Build history of the part. All positions in model axes, mm. A direction names the side the tool comes from. Coordinates: 2 decimals unless noted, no trailing zeros. Loops run counter-clockwise (first coordinate to the right, second up) from the corner with the lowest first, then second, coordinate; pieces in that order, holes last.
Item 1: 3-axis set-ups, long thin cutter, end or side, ignore diameter. For faces 5 (the face through (36.42, -54.31, -4.31)), 6 (the face through (-47.44, -54.53, -50.96)), 7 (the face through (45, -52.5, -28)), 8 (the face through (36.42, -54.31, -51.69)), 9 (the face through (-25.3, -54.74, -27.7)): which of +Z, -Z, +X, -X, +Y, -Y reach the whole face in a straight line?
Item 2: Cut at A-A (x = 0). List the corners of the cut face in (y, z).
Item 3: Mould opens along Z. For faces 1 (the face through (2, -1, 5)), 2 (the face through (25.53, -54.81, -27.7)), 3 (the face through (0, -52, -47.5)), 4 (the face through (0, -52, -8.5)) say: released by +Z, released by -Z, zero draft, split by the parting line, or undercut.
Item 4: Drill centre lines: line 1 along Z through (x, y) = (-49.75, -53.45); line 2 along Z through (x, y) = (49, -55); line 3 along Z through (x, y) = (-0.5, -9.5). Where is each one in solid material? Low to high.
Item 5: Cut at C-C (z = -73). List the corners of the cut face in (x, y), and give its area (3 significant figures).
Item 6: Flat gauge pins, fed straight in: pin 1 (1.5 mm diameter, centred on y = -29, z = -39.5, fed in from +X); pin 2 (10 mm diameter, centred on x = 0.5, y = -53, fed in from -Z); pin 3 (10 mm diameter, centred on x = 6, y = -51, fed in from +Z). Where does each tip first touch, or does it go through?
Item 7: Cut at B-B (z = -39). List the corners of the cut face in (x, y), and give its area (3 significant figures).
from build123d import *

# Parameters (mm, degrees)
SKETCH1_R           = 50.5
BOSS_EXTRUDE1_DEPTH = 76
SKETCH2_R           = 4
BOSS_EXTRUDE2_DEPTH = 27.5
SKETCH3_R           = 15.5
BOSS_EXTRUDE3_DEPTH = 56
CUT_EXTRUDE1_DEPTH  = 14
SKETCH6_R           = 50.5
BOSS_EXTRUDE4_DEPTH = 69
CUT_EXTRUDE2_REACH  = 109
SKETCH7_R           = 2.5
CUT_EXTRUDE3_START  = -229.584638372
SKETCH8_W           = 6
SKETCH8_H           = 2
CUT_EXTRUDE3_DEPTH  = 230.584638372
CIRPATTERN1_COUNT   = 2
CIRPATTERN1_ANGLE   = 90


with BuildPart() as part:
    # Sketch1 → Boss-Extrude1 (new body)
    with BuildSketch(Plane.XY):
        Circle(SKETCH1_R)
    extrude(amount=-BOSS_EXTRUDE1_DEPTH)

    # Sketch2 → Boss-Extrude2 (add)
    with BuildSketch(Plane.XY):
        Circle(SKETCH2_R)
    extrude(amount=BOSS_EXTRUDE2_DEPTH)

    # Sketch3 → section 1 of loft1
    with BuildSketch(Plane(origin=(0, 0, -82), x_dir=(-1, 0, 0), z_dir=(0, 0, -1)), mode=Mode.PRIVATE) as loft1_s1:
        Circle(SKETCH3_R)
    # loft from a face of the part (loft1)
    loft([part.faces().sort_by_distance((0, 0, -76))[0], loft1_s1.sketch])

    # Sketch4 → Boss-Extrude3 (add)
    with BuildSketch(Plane.XY):
        with BuildLine():
            Line((-55.75, -52.5), (-33.867548492, -52.5))
            ThreePointArc((-33.867548492, -52.5), (-25.666216724, -50.654640627), (-18.012227442, -47.178487286))
            ThreePointArc((-18.012227442, -47.178487286), (0, -50.5), (18.012227442, -47.178487286))
            ThreePointArc((18.012227442, -47.178487286), (25.666216724, -50.654640627), (33.867548492, -52.5))
            Line((33.867548492, -52.5), (55.75, -52.5))
            ThreePointArc((55.75, -52.5), (57.75, -54.5), (55.75, -56.5))
            Line((55.75, -56.5), (33.635158839, -56.5))
            ThreePointArc((33.635158839, -56.5), (25.41686368, -54.776707383), (17.660730448, -51.559175711))
            ThreePointArc((17.660730448, -51.559175711), (0, -54.5), (-17.660730448, -51.559175711))
            ThreePointArc((-17.660730448, -51.559175711), (-25.41686368, -54.776707383), (-33.635158839, -56.5))
            Line((-33.635158839, -56.5), (-55.75, -56.5))
            ThreePointArc((-55.75, -56.5), (-57.75, -54.5), (-55.75, -52.5))
        make_face()
    extrude(amount=-BOSS_EXTRUDE3_DEPTH)

    # Sketch5 → Cut-Extrude1 (cut)
    with BuildSketch(Plane.XZ.offset(56.5)):
        Polygon((-31, -8.5), (31, -8.5), (42, 0), (-42, 0), align=None)
        Polygon((-42, -56), (-31, -47.5), (31, -47.5), (42, -56), align=None)
    extrude(amount=-CUT_EXTRUDE1_DEPTH, mode=Mode.SUBTRACT)

    # Sketch6 → Boss-Extrude4 (add)
    with BuildSketch(Plane.XY):
        Circle(SKETCH6_R)
    extrude(amount=-BOSS_EXTRUDE4_DEPTH)

    # Sketch7 → Cut-Extrude2 (cut, up to next)
    with BuildSketch(Plane.XZ.offset(56.5), mode=Mode.PRIVATE) as cut_extrude2_sk1:
        with Locations((-49.75, -6)):
            Circle(SKETCH7_R)
    cut_extrude2_tool1 = extrude(cut_extrude2_sk1.sketch, amount=-CUT_EXTRUDE2_REACH, mode=Mode.PRIVATE) & part.part
    add(cut_extrude2_tool1.solids().sort_by_distance((-49.75, -56.5, -6))[0], mode=Mode.SUBTRACT)
    # Sketch7 → Cut-Extrude2 (cut, up to next)
    with BuildSketch(Plane.XZ.offset(56.5), mode=Mode.PRIVATE) as cut_extrude2_sk2:
        with Locations((-49.75, -50)):
            Circle(SKETCH7_R)
    cut_extrude2_tool2 = extrude(cut_extrude2_sk2.sketch, amount=-CUT_EXTRUDE2_REACH, mode=Mode.PRIVATE) & part.part
    add(cut_extrude2_tool2.solids().sort_by_distance((-49.75, -56.5, -50))[0], mode=Mode.SUBTRACT)
    # Sketch7 → Cut-Extrude2 (cut, up to next)
    with BuildSketch(Plane.XZ.offset(56.5), mode=Mode.PRIVATE) as cut_extrude2_sk3:
        with Locations((49.75, -50)):
            Circle(SKETCH7_R)
    cut_extrude2_tool3 = extrude(cut_extrude2_sk3.sketch, amount=-CUT_EXTRUDE2_REACH, mode=Mode.PRIVATE) & part.part
    add(cut_extrude2_tool3.solids().sort_by_distance((49.75, -56.5, -50))[0], mode=Mode.SUBTRACT)
    # Sketch7 → Cut-Extrude2 (cut, up to next)
    with BuildSketch(Plane.XZ.offset(56.5), mode=Mode.PRIVATE) as cut_extrude2_sk4:
        with Locations((49.75, -6)):
            Circle(SKETCH7_R)
    cut_extrude2_tool4 = extrude(cut_extrude2_sk4.sketch, amount=-CUT_EXTRUDE2_REACH, mode=Mode.PRIVATE) & part.part
    add(cut_extrude2_tool4.solids().sort_by_distance((49.75, -56.5, -6))[0], mode=Mode.SUBTRACT)

    # Sketch8 → Cut-Extrude3 (cut)
    with BuildSketch(Plane(origin=(170.834638372, -107.162802213, -173.5), x_dir=(0, 0, -1), z_dir=(1, 0, 0)).offset(CUT_EXTRUDE3_START)):
        with Locations((-178.5, 110.162802213)):
            Rectangle(SKETCH8_W, SKETCH8_H)
    cut_extrude3 = extrude(amount=CUT_EXTRUDE3_DEPTH, mode=Mode.SUBTRACT)

    # CirPattern1: Cut-Extrude3 ×2 about axis
    cirpattern1_axis = Axis((0, 0, 27.5), (0, 0, -1))
    for i in range(1, CIRPATTERN1_COUNT):
        add(cut_extrude3.rotate(cirpattern1_axis, i * CIRPATTERN1_ANGLE / (CIRPATTERN1_COUNT - 1)), mode=Mode.SUBTRACT)


solid = part.part
Filled sheet:
1. face 5: +Z, -Y
1. face 6: -Y
1. face 7: +Z, -Z, +X
1. face 8: -Z, -Y
1. face 9: +Z, -Z, -Y
2. outline: (-54.5, -47.5) - (-50.5, -47.5) - (-50.5, -76) - (-15.5, -82) - (15.5, -82) - (50.5, -76) - (50.5, 0) - (4, 0) - (4, 2) - (2, 2) - (2, 8) - (4, 8) - (4, 27.5) - (-4, 27.5) - (-4, 0) - (-50.5, 0) - (-50.5, -8.5) - (-54.5, -8.5) - close
3. face 1: undercut
3. face 2: zero draft
3. face 3: released by -Z
3. face 4: released by +Z
4. line 1: z = -56 to -52.5, -47.5 to -8.5, -3.5 to 0
4. line 2: z = -56 to -52.38, -47.62 to -8.38, -3.62 to 0
4. line 3: z = -82 to 0
5. outline: circle Ø101 at (0, 0)
5. area: 8,010 mm2
6. pin 1: stops at x = 41.86
6. pin 2: stops at z = -76.43
6. pin 3: stops at z = 0
7. outline: (-55.75, -56.5) - (-33.64, -56.5) arc R45.08 ccw to (-17.66, -51.56) arc R54.5 ccw to (17.66, -51.56) arc R45.08 ccw to (33.64, -56.5) - (55.75, -56.5) arc R2 ccw to (55.75, -52.5) - (33.87, -52.5) arc R41.08 cw to (18.01, -47.18) arc R50.5 ccw (long way) to (-18.01, -47.18) arc R41.08 cw to (-33.87, -52.5) - (-55.75, -52.5) arc R2 ccw to start
7. area: 8,480 mm2
